from build123d import *

# Parameters (mm, degrees)
SKETCH1_R               = 19.05
EXTRUDE1_DEPTH          = 16.637
SKETCH4_R               = 34.925
EXTRUDE2_DEPTH          = 12.7
SKETCH6_R               = 57.15
EXTRUDE3_DEPTH          = 17.526
CUT_EXTRUDE1_DEPTH      = 102.285505755
CUT_EXTRUDE1_DEPTH_BACK = 102.285505755
SKETCH7_R               = 17.399
SKETCH8_R               = 3.3655
CUT_EXTRUDE2_DEPTH      = 12.7
CIRPATTERN1_COUNT       = 6
SKETCH9_R               = 4.2164
CUT_EXTRUDE3_DEPTH      = 17.526
CIRPATTERN2_COUNT       = 8


with BuildPart() as part:
    # Sketch1 → Extrude1 (new, symmetric)
    with BuildSketch(Plane(origin=(0, 0, 0), x_dir=(1, 0, 0), z_dir=(0, 1, 0))):
        with Locations(Location((0, 0, 0), (0, 0, 270))):
            Circle(SKETCH1_R)
    extrude(amount=EXTRUDE1_DEPTH, both=True)

    # Sketch4 → Extrude2 (add)
    with BuildSketch(Plane(origin=(0, 16.637, 0), x_dir=(-1, 0, 0), z_dir=(0, 1, 0))):
        with Locations(Location((0, 0, 0), (0, 0, 90))):
            Circle(SKETCH4_R)
    extrude(amount=EXTRUDE2_DEPTH)

    # Sketch6 → Extrude3 (add)
    with BuildSketch(Plane.XZ.offset(16.637)):
        with Locations(Location((12.7, 0, 0), (0, 0, 270))):
            Circle(SKETCH6_R)
    extrude(amount=EXTRUDE3_DEPTH)

    # Sketch7 → Cut-Extrude1 (cut, two sides: drawn at the far end of the back side and taken through both)
    with BuildSketch(Plane.XZ.offset(16.637).offset(-CUT_EXTRUDE1_DEPTH_BACK)):
        with Locations(Location((0, 0, 0), (0, 0, 270))):
            Circle(SKETCH7_R)
    extrude(amount=CUT_EXTRUDE1_DEPTH + CUT_EXTRUDE1_DEPTH_BACK, mode=Mode.SUBTRACT)

    # Sketch8 → Cut-Extrude2 (cut)
    with BuildSketch(Plane(origin=(0, 16.637, 0), x_dir=(-1, 0, 0), z_dir=(0, 1, 0))):
        with Locations(Location((0, 29.337, 0), (0, 0, 90))):
            Circle(SKETCH8_R)
    cut_extrude2 = extrude(amount=CUT_EXTRUDE2_DEPTH, mode=Mode.SUBTRACT)

    # CirPattern1: Cut-Extrude2 ×6 about axis
    cirpattern1_axis = Axis((0, 0, 0), (0, 1, 0))
    for i in range(1, CIRPATTERN1_COUNT):
        add(cut_extrude2.rotate(cirpattern1_axis, i * 360 / CIRPATTERN1_COUNT), mode=Mode.SUBTRACT)

    # Sketch9 → Cut-Extrude3 (cut)
    with BuildSketch(Plane.XZ.offset(16.637)):
        with Locations((12.7, 46.101)):
            Circle(SKETCH9_R)
    cut_extrude3 = extrude(amount=CUT_EXTRUDE3_DEPTH, mode=Mode.SUBTRACT)

    # CirPattern2: Cut-Extrude3 ×8 about axis
    cirpattern2_axis = Axis((12.7, 0, 0), (0, 1, 0))
    for i in range(1, CIRPATTERN2_COUNT):
        add(cut_extrude3.rotate(cirpattern2_axis, i * 360 / CIRPATTERN2_COUNT), mode=Mode.SUBTRACT)


solid = part.part
CAD build for the part. Positions are in the model's coordinates, mm. A direction names the side the tool comes from. Coordinates: 2 decimals unless noted, no trailing zeros. Write each loop counter-clockwise with the first axis right and the second up, starting at its lowest first coordinate (ties: lowest second). Pieces come first, ordered by that corner, then holes. Notation, with made-up numbers: (-35.5, -34.5) - (12.5, -34.5) arc R22 cw to (12.5, -0.5) - close; hole circle Ø9 at (18.25, 4.5). An arc over 180 degrees is marked (long way). Use a Markdown table: item, result. Add a question column.
Item 1: Drill centre lines: L1, parallel to X at y = -19, z = 0; L2, parallel to Y at x = 4.5, z = 31; L3, parallel to Y at x = -34, z = 2. Where is each one in solid material? Low to high. Write a range as from..to.
Item 2: Band-saw the part on A-A, the plane z = 0. Give the cut face in (x, y) (3 decimals).
Item 3: Band-saw the part on C-C, the plane x = 45. Give the cut face in (y, z).
Item 4: Band-saw the part on B-B, the plane x = 12.7. Give the cut face in (y, z), and give its area (3 significant figures).
Item 5: Band-saw the part on D-D, the plane y = -13.5. Give the cut face in (x, z).
Item 6: 3-axis set-ups, long thin cutter, end or side, ignore diameter. For faces 1 (the face through (25.26, 22.9, 18.03)), 2 (the face through (-37.58, -25.28, -0.55)), 3 (the face through (-15, 16.637, 15)): which of +Z, -Z, +X, -X, +Y, -Y reach the whole face in a straight line?
Item 7: Flat gauge pins, fed straight in: pin 1 (4 mm diameter, centred on x = -25.41, z = -14.67, fed in from +Y); pin 2 (21 mm diameter, centred on x = 3.5, z = -2.5, fed in from -Y); pin 3 (2 mm diameter, centred on x = -31.5, y = -18, fed in from -Z) (3 decimals); pin 4 (10 mm diameter, centred on y = 7.5, z = -22.5, fed in from -X). Where does each tip first touch, or does it go through?
Item 8: Mould opens along Y. For faces 4 (the face through (-11.59, 0.23, -15.12)), 5 (the face through (26, -16.637, 1)), 6 (the face through (41.278, -25.277, -31.329)), 7 (the face through (26, -34.163, 1)) say: pulls with the +Y half, pulls with the -Y half, needs draft (parallel to the pull), parting line crosses it, or undercut.
Numbers:
| question | item | result |
|---|---|---|
| 1 | L1 | -44.45..-37.62, -29.18..-17.4, 17.4..54.58, 63.02..69.85 |
| 1 | L2 | -34.16..-16.64, 16.64..29.34 |
| 1 | L3 | 16.64..29.34 |
| 2 | outline | (-44.45, -34.163) - (-37.617, -34.163) - (-37.617, -16.637) - (-44.45, -16.637) - close; (-34.925, 16.637) - (-19.05, 16.637) - (-19.05, -16.637) - (-29.185, -16.637) - (-29.185, -34.163) - (-17.399, -34.163) - (-17.399, 29.337) - (-34.925, 29.337) - close; (17.399, -34.163) - (54.585, -34.163) - (54.585, -16.637) - (19.05, -16.637) - (19.05, 16.637) - (34.925, 16.637) - (34.925, 29.337) - (17.399, 29.337) - close; (63.017, -34.163) - (69.85, -34.163) - (69.85, -16.637) - (63.017, -16.637) - close |
| 3 | outline | (-34.16, -47.15) - (-16.64, -47.15) - (-16.64, -36.8) - (-34.16, -36.8) - close; (-34.16, -28.39) - (-16.64, -28.39) - (-16.64, 28.39) - (-34.16, 28.39) - close; (-34.16, 36.8) - (-16.64, 36.8) - (-16.64, 47.15) - (-34.16, 47.15) - close |
| 4 | outline | (-34.16, -57.15) - (-16.64, -57.15) - (-16.64, -50.32) - (-34.16, -50.32) - close; (-34.16, -41.88) - (-16.64, -41.88) - (-16.64, -14.2) - (16.64, -14.2) - (16.64, -32.53) - (29.34, -32.53) - (29.34, -11.89) - (-34.16, -11.89) - close; (-34.16, 11.89) - (29.34, 11.89) - (29.34, 32.53) - (16.64, 32.53) - (16.64, 14.2) - (-16.64, 14.2) - (-16.64, 41.88) - (-34.16, 41.88) - close; (-34.16, 50.32) - (-16.64, 50.32) - (-16.64, 57.15) - (-34.16, 57.15) - close |
| 4 | area | 1,970 mm2 |
| 5 | outline | circle Ø38.1 at (0, 0); hole circle Ø34.8 at (0, 0) |
| 6 | face 1 | +Y |
| 6 | face 2 | -Y |
| 6 | face 3 | none |
| 7 | pin 1 | y = -16.64 |
| 7 | pin 2 | through |
| 7 | pin 3 | z = -37.415 |
| 7 | pin 4 | x = -7.53 |
| 8 | face 4 | undercut |
| 8 | face 5 | undercut |
| 8 | face 6 | needs draft |
| 8 | face 7 | pulls with the -Y half |
